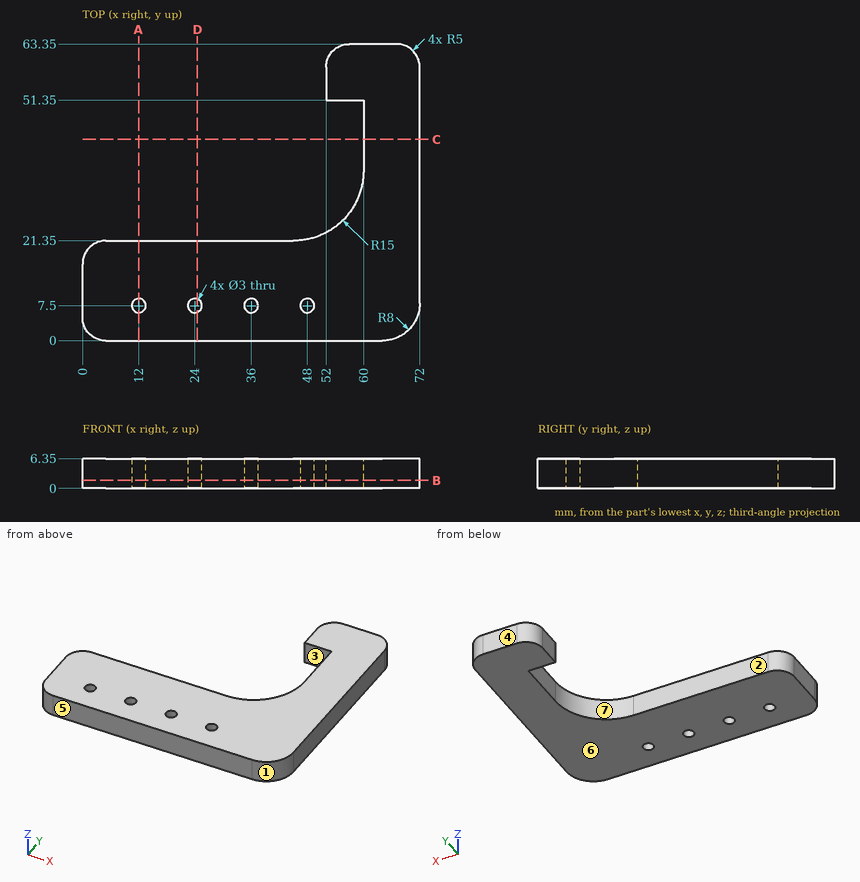
Job drawing, mm, ordinate dimensions from the low corner. One solid piece. A direction names the side the tool comes from. Coordinates: 2 decimals unless noted, no trailing zeros. Write each loop counter-clockwise with the first axis right and the second up, starting at its lowest first coordinate (ties: lowest second). Pieces come first, ordered by that corner, then holes.
Item 1: Pin check, flat tip, straight feed: pin 1 (1.9 mm diameter, centred on y = 54, z = 2, fed in from -X). Stop position of the tip, or through.
Item 2: Which spindle directions (+Z, -Z, +X, -X, +Y, -Y) get a long thin tool onto all of the face, cutting with end or side? Do the marked faces 1, 2 and 3. Say none if no direction does.
Item 3: Slice it at D-D (x = 24.5). Write the cut outline in (y, z).
Item 4: Slice it at C-C (y = 43). Write the cut outline in (x, z).
Item 5: Slice it at A-A (x = 12). Write the cut outline in (y, z).
Item 6: Slice it at B-B (z = 1.75). Write the cut outline in (x, y).
Item 7: Mould opens along Y. For the marked faces 4, 5, 6 and 7 say: released by +Y, released by -Y, zero draft, split by the parting line, or undercut.
Item 8: Probe line 1 (Y direction, x = 36, z = 2); line 2 (Y direction, x = 48, z = 5.25); line 3 (Y direction, x = 5, z = 1). List the from-to ranges inside material, lowest first.
Results found:
1. pin 1: stops at x = 52
2. face 1: +Z, -Z, +X, -Y
2. face 2: +Z, -Z, -X, +Y
2. face 3: +Z, -Z, -X
3. outline: (0, 0) - (6.09, 0) - (6.09, 6.35) - (0, 6.35) - close; (8.91, 0) - (21.35, 0) - (21.35, 6.35) - (8.91, 6.35) - close
4. outline: (60, 0) - (72, 0) - (72, 6.35) - (60, 6.35) - close
5. outline: (0, 0) - (6, 0) - (6, 6.35) - (0, 6.35) - close; (9, 0) - (21.35, 0) - (21.35, 6.35) - (9, 6.35) - close
6. outline: (0, 5) arc R5 ccw to (5, 0) - (64, 0) arc R8 ccw to (72, 8) - (72, 58.35) arc R5 ccw to (67, 63.35) - (57, 63.35) arc R5 ccw to (52, 58.35) - (52, 51.35) - (60, 51.35) - (60, 36.35) arc R15 cw to (45, 21.35) - (5, 21.35) arc R5 ccw to (0, 16.35) - close; hole circle Ø3 at (12, 7.5); hole circle Ø3 at (24, 7.5); hole circle Ø3 at (36, 7.5); hole circle Ø3 at (48, 7.5)
7. face 4: released by +Y
7. face 5: released by -Y
7. face 6: zero draft
7. face 7: undercut
8. line 1: y = 0 to 6, 9 to 21.35
8. line 2: y = 0 to 6, 9 to 21.65
8. line 3: y = 0 to 21.35
